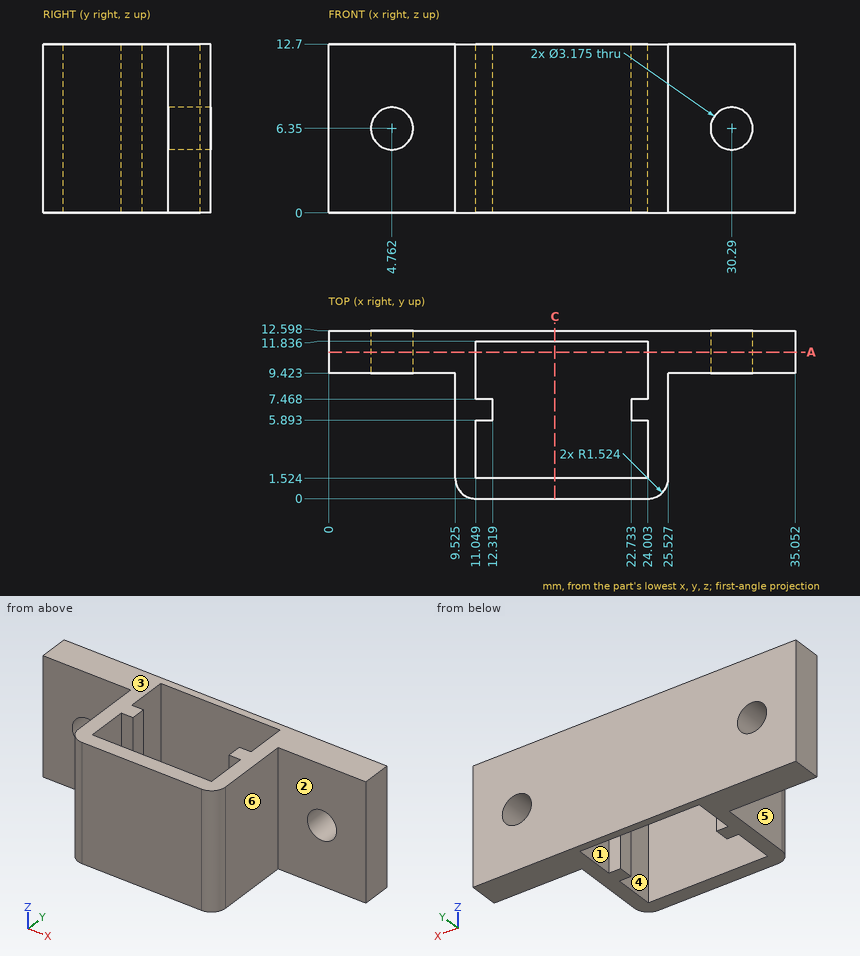
Here's the drawing with two shaded views (mm, measured from the low corner). I have some questions. A direction names the side the tool comes from. Give positions to 0.01 mm unless a question says otherwise; leave off trailing zeros. Order: outer loops, then holes, each group sorted by start corner. A loop starts at its lowest first (then second) coordinate and runs counter-clockwise, first axis right, second up. Notation, with made-up numbers: M -0.75,-30 L 49.25,-30 A19 cw 49.25,-16 Z; hole C 38.5,-32.5 d2. An arc over 180 degrees is marked long. Answer as a JSON object with one key per item and string values. Group by question number.
1) On a 3-axis mill with a long thin cutter (end or side, diameter ignored), from which of +Z, -Z, +X, -X, +Y, -Y can I reach the whole of each face in a straight line? I mean the marked faces 4, 5 and 6. Say none if no direction works.
2) I'm going to push flat-ended pins straight in: pin 1 Ø0.5 at (y, z) = (6.5, 5) entering from +X; pin 2 Ø3 at (y, z) = (6.5, 5.5) entering from -X (1 decimal); pin 3 Ø1.5 at (x, z) = (6.5, 6) entering from -Y; pin 4 Ø1.9 at (x, z) = (4.76, 6.35) entering from -Y. Where does each tip first touch, or does it pass through?
3) Suppose I cut it at C-C, the plane x = 17. Write out the boundary of the cut face in (y, z) (1 decimal).
4) Please list where these lines run through material, in increasing order: L1, parallel to X at y = 10.5, z = 9.5; L2, parallel to Y at x = 19.5, z = 8.25 (1 decimal); L3, parallel to X at y = 10.75, z = 5.75. Write a range as [from, to].
5) We'd pull the mould along Y, two halves only. Please class the marked faces 1, 2 and 3: pulls with the +Y half, pulls with the -Y half, needs draft (parallel to the pull), parting line crosses it, or undercut.
6) Suppose I cut it at A-A, the plane y = 11. Count the separate pieces of the cut face and the enclosed holes in it, plus the area to 3 significant figures.
Results found:
{
 "1": {"face 4": "+Z, -Z", "face 5": "+Z, -Z, -X, -Y", "face 6": "+Z, -Z, +X, -Y"},
 "2": {"pin 1": "x = 25.53", "pin 2": "x = 9.5", "pin 3": "y = 9.42", "pin 4": "through"},
 "3": {"outline": "M 0,0 L 1.5,0 L 1.5,12.7 L 0,12.7 Z; M 11.8,0 L 12.6,0 L 12.6,12.7 L 11.8,12.7 Z"},
 "4": {"L1": "[0, 11.05], [24, 35.05]", "L2": "[0, 1.5], [11.8, 12.6]", "L3": "[0, 3.29], [6.23, 11.05], [24, 28.82], [31.76, 35.05]"},
 "5": {"face 1": "undercut", "face 2": "pulls with the -Y half", "face 3": "needs draft"},
 "6": {"separate pieces": "2", "enclosed holes": "2", "area": "265 mm²"}
}
